Source: CAD feature listing. Evaluate the final solid. Frame: model axes, mm. Face numbers are marked on the shaded views. Give positions to 0.01 mm unless a question says otherwise; leave off trailing zeros. Loops run counter-clockwise (first coordinate to the right, second up) from the corner with the lowest first, then second, coordinate; pieces in that order, holes last.
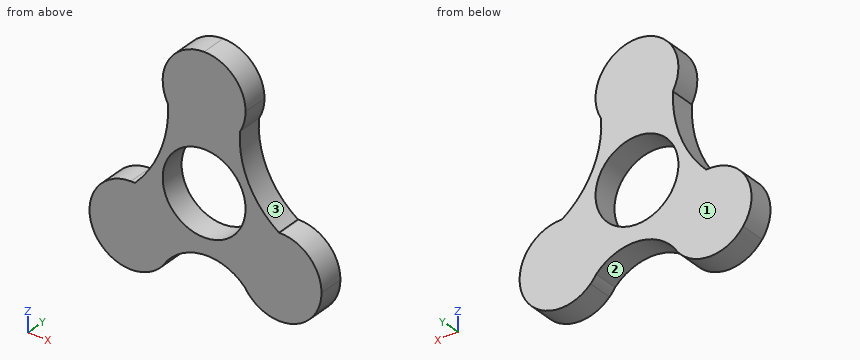
from build123d import *

# Parameters (mm, degrees)
F0_R     = 11.25
F1_DEPTH = 7


with BuildPart() as f1:
    # F0 (on Front) → F1 (new body)
    with BuildSketch(Plane.XZ):
        with BuildLine():
            Line((0, 24.8070023954), (-9.7427857926, 19.1820023954))
            ThreePointArc((-9.7427857926, 19.1820023954), (0, 13.5570023954), (9.7427857926, 19.1820023954))
            Line((9.7427857926, 19.1820023954), (0, 24.8070023954))
        make_face()
        with BuildLine():
            ThreePointArc((0, 36.0570023954), (-9.7427857926, 30.4320023954), (-9.7427857926, 19.1820023954))
            Line((-9.7427857926, 19.1820023954), (0, 24.8070023954))
            Line((0, 24.8070023954), (0, 36.0570023954))
        make_face()
        with BuildLine():
            ThreePointArc((9.7427857926, 19.1820023954), (0, 13.5570023954), (-9.7427857926, 19.1820023954))
            ThreePointArc((-9.7427857926, 19.1820023954), (-11.8794963915, 6.6600701003), (-18.785878025, -4.0013656998))
            ThreePointArc((-18.785878025, -4.0013656998), (-11.5266597843, -7.6312649105), (-8.5989967734, -15.2010209858))
            ThreePointArc((-8.5989967734, -15.2010209858), (-8.9823312276, -18.1127352432), (-10.1062109808, -20.8260209858))
            ThreePointArc((-10.1062109808, -20.8260209858), (0.3044783334, -15.6283312232), (11.0680600024, -20.0491615206))
            ThreePointArc((11.0680600024, -20.0491615206), (10.7001408508, -8.750972982), (20.3337626304, -2.8367731067))
            ThreePointArc((20.3337626304, -2.8367731067), (12.0864921747, 6.7528147477), (9.7427857926, 19.1820023954))
        make_face()
        Circle(F0_R, mode=Mode.SUBTRACT)
        with BuildLine():
            Line((0, 24.8070023954), (9.7427857926, 19.1820023954))
            ThreePointArc((9.7427857926, 19.1820023954), (10.8666655458, 21.895288138), (11.25, 24.8070023954))
            ThreePointArc((11.25, 24.8070023954), (7.9549512883, 32.7619536837), (0, 36.0570023954))
            Line((0, 36.0570023954), (0, 24.8070023954))
        make_face()
        with BuildLine():
            ThreePointArc((-19.8489967734, -5.0313835964), (-19.3113897365, -4.5226166596), (-18.785878025, -4.0013656998))
            ThreePointArc((-18.785878025, -4.0013656998), (-19.3168417059, -3.9636142127), (-19.8489967734, -3.9510209858))
            Line((-19.8489967734, -3.9510209858), (-19.8489967734, -5.0313835964))
        make_face()
        with BuildLine():
            ThreePointArc((-8.5989967734, -15.2010209858), (-11.5266597843, -7.6312649105), (-18.785878025, -4.0013656998))
            ThreePointArc((-18.785878025, -4.0013656998), (-19.3113897365, -4.5226166596), (-19.8489967734, -5.0313835964))
            Line((-19.8489967734, -5.0313835964), (-19.8489967734, -15.2010209858))
            Line((-19.8489967734, -15.2010209858), (-10.1062109808, -20.8260209858))
            ThreePointArc((-10.1062109808, -20.8260209858), (-8.9823312276, -18.1127352432), (-8.5989967734, -15.2010209858))
        make_face()
        with BuildLine():
            ThreePointArc((20.6060428172, -3.0198064633), (20.4695953446, -2.928747042), (20.3337626304, -2.8367731067))
            ThreePointArc((20.3337626304, -2.8367731067), (10.7001408508, -8.750972982), (11.0680600024, -20.0491615206))
            ThreePointArc((11.0680600024, -20.0491615206), (11.8662666045, -20.9755321249), (12.5810078032, -21.9677222755))
            Line((12.5810078032, -21.9677222755), (20.6060428172, -14.0834776685))
            Line((20.6060428172, -14.0834776685), (20.6060428172, -3.0198064633))
        make_face()
        with BuildLine():
            ThreePointArc((20.6060428172, -2.8334776685), (20.4698927529, -2.8343015582), (20.3337626304, -2.8367731067))
            ThreePointArc((20.3337626304, -2.8367731067), (20.4695953446, -2.928747042), (20.6060428172, -3.0198064633))
            Line((20.6060428172, -3.0198064633), (20.6060428172, -2.8334776685))
        make_face()
        with BuildLine():
            Line((-19.8489967734, -5.0313835964), (-19.8489967734, -3.9510209858))
            ThreePointArc((-19.8489967734, -3.9510209858), (-29.9165162791, -10.1803087852), (-28.834973309, -21.9696785855))
            Line((-28.834973309, -21.9696785855), (-19.8489967734, -15.2010209858))
            Line((-19.8489967734, -15.2010209858), (-19.8489967734, -5.0313835964))
        make_face()
        with BuildLine():
            ThreePointArc((31.8560428172, -14.0834776685), (28.5609941056, -6.1285263801), (20.6060428172, -2.8334776685))
            Line((20.6060428172, -2.8334776685), (20.6060428172, -3.0198064633))
            Line((20.6060428172, -3.0198064633), (20.6060428172, -14.0834776685))
            Line((20.6060428172, -14.0834776685), (30.3488286098, -19.7084776685))
            ThreePointArc((30.3488286098, -19.7084776685), (31.472708363, -16.9951919259), (31.8560428172, -14.0834776685))
        make_face()
        with BuildLine():
            ThreePointArc((12.5810078032, -21.9677222755), (11.8662666045, -20.9755321249), (11.0680600024, -20.0491615206))
            ThreePointArc((11.0680600024, -20.0491615206), (11.7722940288, -21.0496374673), (12.5810078032, -21.9677222755))
        make_face()
        with BuildLine():
            ThreePointArc((-28.834973309, -21.9696785855), (-19.1633013314, -26.4301047312), (-10.1062109808, -20.8260209858))
            Line((-10.1062109808, -20.8260209858), (-19.8489967734, -15.2010209858))
            Line((-19.8489967734, -15.2010209858), (-28.834973309, -21.9696785855))
        make_face()
        with BuildLine():
            Line((20.6060428172, -14.0834776685), (12.5810078032, -21.9677222755))
            ThreePointArc((12.5810078032, -21.9677222755), (22.0250965452, -25.2436204327), (30.3488286098, -19.7084776685))
            Line((30.3488286098, -19.7084776685), (20.6060428172, -14.0834776685))
        make_face()
    extrude(amount=F1_DEPTH)


solid = f1.part
1) Cut plane B-B (y = -1). Return loops of the section in (x, z), and give its area (3 significant figures).
Checks:
outline: (-18.79, -4) arc R11.25 ccw (long way) to (-10.11, -20.83) arc R14.07 cw to (11.07, -20.05) arc R11.25 ccw (long way) to (20.33, -2.84) arc R24.42 cw to (9.74, 19.18) arc R11.25 ccw (long way) to (-9.74, 19.18) arc R31.52 cw to start; hole circle Ø22.5 at (0, 0)
area: 1,580 mm2
2) Contact query for flat-ended pins moving along their axis: P1, Ø3, axis at y = -4.5, z = -8, coming from the +X side; P2, Ø10, axis at x = 0.5, z = -4.5, coming from the +Y side; P3, Ø3, axis at x = -19.5, y = -3.5, coming from the +Z side; P4, Ø3, axis at x = -7.5, y = -3.5, coming from the +Z side. Output: stop coordinate, or through.
Checks:
P1: stops at x = 30.88
P2: passes through
P3: stops at z = -3.17
P4: stops at z = 34.32
3) Cut plane D-D (z = 0). Return loops of the section in (x, y), and give its area (3 significant figures).
Checks:
outline: (-15.45, -7) - (-11.25, -7) - (-11.25, 0) - (-15.45, 0) - close; (11.25, -7) - (16.9, -7) - (16.9, 0) - (11.25, 0) - close
area: 68.9 mm2
4) Cut plane C-C (x = 27). Return loops of the section in (y, z).
Checks:
outline: (-7, -23.34) - (0, -23.34) - (0, -4.83) - (-7, -4.83) - close
5) Ray query, probe 1 along Z at (x, y) = (-5, -2); probe 2 along Z at (x, y) = (0, -2); probe 3 along X at (y, z) = (-5.5, -5). Return the intervals inside material, ascending.
Checks:
probe 1: z = -16.88 to -10.08, 10.08 to 34.88
probe 2: z = -15.64 to -11.25, 11.25 to 36.06
probe 3: x = -24.59 to -10.08, 10.08 to 27.24
6) Pull-direction query (X, two-part tool) for the marked faces 1, 2 and 3; classes: released by +X, released by -X, zero draft, split by the parting line, or undercut.
Checks:
face 1: zero draft
face 2: undercut
face 3: released by +X
7) Cut plane A-A (z = 7.5). Return loops of the section in (x, y).
Checks:
outline: (-11.57, -7) - (-8.39, -7) - (-8.39, 0) - (-11.57, 0) - close; (8.39, -7) - (11.74, -7) - (11.74, 0) - (8.39, 0) - close
